Geometry check sheet. Reference: the model listing, model coordinates, mm. A direction names the side the tool comes from. Give positions to 0.01 mm unless a question says otherwise; leave off trailing zeros. Order: outer loops, then holes, each group sorted by start corner. A loop starts at its lowest first (then second) coordinate and runs counter-clockwise, first axis right, second up. Notation, with made-up numbers: M -37,37.25 L -22,37.25 A20 cw -22,48.25 Z; hole C 15.25,28.5 d11. An arc over 180 degrees is marked long. Answer as CSV lines item,"result". Start each with the question number.
```python
from build123d import *

# Parameters (mm, degrees)
SKETCH1_W           = 40
SKETCH1_H           = 20
BOSS_EXTRUDE1_DEPTH = 90
FILLET1_R           = 1
SKETCH2_R           = 15
CUT_EXTRUDE1_DEPTH  = 10
FILLET2_R           = 6.3


with BuildPart() as part:
    # Sketch1 → Boss-Extrude1 (new body)
    with BuildSketch(Plane.XY):
        Rectangle(SKETCH1_W, SKETCH1_H)
    extrude(amount=BOSS_EXTRUDE1_DEPTH)

    # Fillet1
    fillet1_edges = [part.edges().sort_by_distance(p)[0] for p in [
        (20, -10, 45),
        (-20, -10, 45),
    ]]
    fillet(fillet1_edges, radius=FILLET1_R)

    # Sketch2 → Cut-Extrude1 (cut)
    with BuildSketch(Plane(origin=(0, 10, 0), x_dir=(1, 0, 0), z_dir=(0, 1, 0))):
        with Locations(Location((0, -45, 0), (0, 0, 270))):
            Circle(SKETCH2_R)
    extrude(amount=-CUT_EXTRUDE1_DEPTH, mode=Mode.SUBTRACT)

    # Fillet2
    # the kernel refuses this fillet: 6.3 mm, written as the material it takes off along each edge
    with BuildSketch(Plane(origin=(-20, 10, -15.75), x_dir=(0, -1, 0), z_dir=(0, 0, 1))) as fillet2_piece_1:
        with BuildLine():
            CenterArc((FILLET2_R, FILLET2_R), FILLET2_R, 180, 90)
            Line((0, FILLET2_R), (0, 0))
            Line((0, 0), (FILLET2_R, 0))
        make_face()
    extrude(amount=121.5, mode=Mode.SUBTRACT)
    with BuildSketch(Plane(origin=(20, 10, -15.75), x_dir=(0, -1, 0), z_dir=(0, 0, 1))) as fillet2_piece_2:
        with BuildLine():
            CenterArc((FILLET2_R, -FILLET2_R), FILLET2_R, 90, 90)
            Line((0, -FILLET2_R), (0, 0))
            Line((0, 0), (FILLET2_R, 0))
        make_face()
    extrude(amount=121.5, mode=Mode.SUBTRACT)


solid = part.part
```
Item 1: Section check A-A on y = 1.25. Record the boundary of the cut face in (x, z).
Item 2: Section check D-D on z = 49. Record the boundary of the cut face in (x, y), then the cut area to 3 significant figures.
Item 3: Scan lines: line 1 along X through (y, z) = (4, 45); line 2 along Z through (x, y) = (0, 7.5); line 3 along Y through (x, z) = (-14, 47). Record each from-to range of solid material in increasing order.
Item 4: Depth check by flat-ended pin: pin 1 Ø15 at (x, z) = (6, 43.5) entering from +Y. Enter the tip coordinate at first touch or a pass-through.
Item 5: Section check B-B on x = 9. Record the boundary of the cut face in (y, z), then the cut area to 3 significant figures.
Item 6: Access from +Z, -Z, +X, -X, +Y, -Y to the whole of each face (thin tool, end or side, straight path). Record for faces 1 (the face through (0.66, 5.07, 30.015)), 2 (the face through (-20, -3, 44)).
Item 7: Section check C-C on z = 64. Record the boundary of the cut face in (x, y).
Numbers:
1,outline,"M -20,0 L 20,0 L 20,90 L -20,90 Z; hole C 0,45 d30"
2,outline,"M -20,-9 A1 ccw -19,-10 L 19,-10 A1 ccw 20,-9 L 20,3.7 A6.3 ccw 14.46,9.95 L 14.46,0 L -14.46,0 L -14.46,9.95 A6.3 ccw -20,3.7 Z"
2,area,"493 mm2"
3,line 1,"-19.99 to -15, 15 to 19.99"
3,line 2,"0 to 30, 60 to 90"
3,line 3,"-10 to 0"
4,pin 1,"y = 0"
5,outline,"M -10,0 L 10,0 L 10,33 L 0,33 L 0,57 L 10,57 L 10,90 L -10,90 Z"
5,area,"1,560 mm2"
6,face 1,"+Y"
6,face 2,"+Z, -Z, -X, +Y, -Y"
7,outline,"M -20,-9 A1 ccw -19,-10 L 19,-10 A1 ccw 20,-9 L 20,3.7 A6.3 ccw 13.7,10 L -13.7,10 A6.3 ccw -20,3.7 Z"
